Here's how the part is built. I have some questions about the finished solid (model axes, mm). A direction names the side the tool comes from. Round coordinates to 2 decimals unless told otherwise and drop trailing zeros. Loops run counter-clockwise (first coordinate to the right, second up) from the corner with the lowest first, then second, coordinate; pieces in that order, holes last. Notation, with made-up numbers: M 69,49 L 114,49 A29 cw 114,81 Z; hole C 1.5,36.5 d8. An arc over 180 degrees is marked long. Answer as a JSON object with one key per item and string values.
Autodesk Inventor part; units mm, degrees
ref_plane "YZ Plane" through (0, 0, 0) normal (1, 0, 0) x (0, 1, 0)
ref_plane "XZ Plane" through (0, 0, 0) normal (0, 1, 0) x (-1, 0, 0)
ref_plane "XY Plane" through (0, 0, 0) normal (0, 0, 1) x (1, 0, 0)
sketch "Boceto1" plane through (0, 0, 0) normal (1, 0, 0) x (0, 1, 0)
  circle A0 centre (0, 0) radius 2.9
  line L0 (0, 5) -> (0, 5)
  line L1 (5, 0) -> (5, 0)
  line L2 (0, -5) -> (0, -5)
  line L3 (-5, 0) -> (-5, 0)
  circle A1 centre (0, 0) radius 4
  dimension "d0" = 5.8
  dimension "d11" = 8
extrude "Extrusión1" add sketch "Boceto1" along normal blind 5
sketch "Boceto2" plane through (5, 0, 0) normal (1, 0, 0) x (0, 0, -1)
  line L0 (1.1, -2.6) -> (-1.1, -2.6)
  line L1 (-1.1, -2.6) -> (-1.1, 2.6)
  line L2 (-1.1, 2.6) -> (1.1, 2.6)
  line L3 (1.1, 2.6) -> (1.1, -2.6)
  line L4 (1.1, -2.6) -> (-1.1, 2.6)
  line L5 (-1.1, -2.6) -> (1.1, 2.6)
  line L6 (2.6, -1.1) -> (-2.6, -1.1)
  line L7 (-2.6, -1.1) -> (-2.6, 1.1)
  line L8 (-2.6, 1.1) -> (2.6, 1.1)
  line L9 (2.6, 1.1) -> (2.6, -1.1)
  line L10 (2.6, -1.1) -> (-2.6, 1.1)
  line L11 (-2.6, -1.1) -> (2.6, 1.1)
  circle A0 centre (0, 0) radius 1.6
  circle A1 centre (0, 0) radius 4
  circle A2 centre (0, 0) radius 4
  point P0 (-1.1, -1.1619)
  point P1 (-1.1619, -1.1)
  point P2 (-1.1619, 1.1)
  point P3 (-1.1, 1.1619)
  point P4 (1.1, 1.1619)
  point P5 (1.1619, 1.1)
  point P6 (1.1619, -1.1)
  point P7 (1.1, -1.1619)
  dimension "d6" = 2.2
  dimension "d7" = 5.2
  dimension "d8" = 3.2
extrude "Extrusión2" add sketch "Boceto2" along normal blind 7
properties part number "AcopleMotor"
Item 1: For faces 1 (the face through (5, -1.3, -1.3)), 2 (the face through (12, -2, -2)), 3 (the face through (8, 2, 1.1)), which set-ups out of +Z, -Z, +X, -X, +Y, -Y let a thin tool reach every point of the face, with its end or its side?
Solution:
{"face 1": "-X", "face 2": "+Z, -Z, +X, +Y, -Y", "face 3": "+X, -X"}
Item 2: If I drill on L1, parallel to Z at x = 2.4, y = 0; L2, parallel to Z at x = 4.5, y = 1.25; L3, parallel to Y at x = 9.5, z = -2.5, over which ranges is the centre line in solid material (lowest first)? Write a range as from..to.
Solution:
{"L1": "z = -4..-2.9, 2.9..4", "L2": "z = -3.8..-2.62, 2.62..3.8", "L3": "y = -3.12..-1.1, 1.1..3.12"}
Item 3: I want a section at B-B on z = 0. List the corners of the cut face in (x, y) for me, plus the area to 3 significant figures.
Solution:
{"outline": "M 0,-4 L 12,-4 L 12,-2.6 L 5,-2.6 L 5,-2.9 L 0,-2.9 Z; M 0,2.9 L 5,2.9 L 5,2.6 L 12,2.6 L 12,4 L 0,4 Z", "area": "30.6 mm2"}
Item 4: For P1, Ø1.7, axis at y = -0.5, z = -1, coming from the -X side; P2, Ø1.6, axis at x = 7, z = -2, coming from the -Y side; P3, Ø0.7, axis at x = 10, y = 1.5, coming from the -Z side, each with a flat end and sliding along its axis, tell me the tip position at first contact or that it passes through.
Solution:
{"P1": "stops at x = 5", "P2": "stops at y = -3.82", "P3": "stops at z = -3.83"}
Item 5: I want a section at A-A on x = 7.5. List the corners of the cut face in (y, z) for me.
Solution:
{"outline": "C 0,0 d8; hole M -2.6,-1.1 L -1.16,-1.1 A1.6 ccw -1.1,-1.16 L -1.1,-2.6 L 1.1,-2.6 L 1.1,-1.16 A1.6 ccw 1.16,-1.1 L 2.6,-1.1 L 2.6,1.1 L 1.16,1.1 A1.6 ccw 1.1,1.16 L 1.1,2.6 L -1.1,2.6 L -1.1,1.16 A1.6 ccw -1.16,1.1 L -2.6,1.1 Z"}
Item 6: I want a section at D-D on x = 4.5. List the corners of the cut face in (y, z) for me, plus the area to 3 significant figures.
Solution:
{"outline": "C 0,0 d8; hole C 0,0 d5.8", "area": "23.8 mm2"}
Item 7: We'd pull the mould along Z, two halves only. Please class faces 4 (the face through (0, 3, 1)), 5 (the face through (4.58, 3.71, -1.49)), 6 (the face through (8, 1.1, -2)): +Z half, -Z half, draft (parallel to the pull), parting line (faces both ways), or undercut.
Solution:
{"face 4": "draft", "face 5": "parting line", "face 6": "undercut"}
